Model file for the job. Use its own axes, mm. A direction names the side the tool comes from. Coordinates: 2 decimals unless noted, no trailing zeros. Write each loop counter-clockwise with the first axis right and the second up, starting at its lowest first coordinate (ties: lowest second). Pieces come first, ordered by that corner, then holes. Notation, with made-up numbers: M -36.5,27 L -22.5,27 A29 cw -22.5,64 Z; hole C 29.25,59 d4. An arc over 180 degrees is marked long. Put each result on its own line as item: value. Start each with the question number.
Q1. Which spindle directions (+Z, -Z, +X, -X, +Y, -Y) get a long thin tool onto all of the face, cutting with end or side? Do faces 1 (the flat face through (-58, -588, 85.706)), 2 (the flat face through (-38.133, -588, 26)), 3 (the flat face through (-80.633, -588, 26)). Say none if no direction does.
Q2. Pull direction Z, two halves, no side cores. Call faces 4 (the flat face through (-82.133, -588, 54)), 5 (the flat face through (-59, -588, -34.294)), 6 (the flat face through (-36.633, -588, 26)), 7 (the flat face through (-83.633, -588, 54)): pulls with the +Z half, pulls with the -Z half, needs draft (parallel to the pull), parting line crosses it, or undercut.
Q3. Drill centre lines: line 1 along X through (y, z) = (-846, 78.5); line 2 along X through (y, z) = (-259, 49); line 3 along Z through (x, y) = (-53.5, -513). Where is each one in solid material? Low to high.
Q4. Cut at A-A (x = -58.5). Write the cut outline in (y, z), then the cut area to 3 significant figures.
Q5. Drop flat-ended pins along their axis: pin 1 (5 mm diameter, centred on y = -998.5, z = -21.5, fed in from +X); pin 2 (4 mm diameter, centred on y = -742, z = 70.5, fed in from +X); pin 3 (19 mm diameter, centred on y = -639, z = 21, fed in from +X). Give the stop position or say it passes through.
```python
from build123d import *

# Parameters (mm, degrees)
F1_DEPTH = 1192
F2_T     = -1.5


with BuildPart() as f1:
    # F0 (on Front) → F1 (new body)
    with BuildSketch(Plane.XZ):
        with BuildLine():
            Line((-40.846474, 85.706456), (-76.418904, 85.706456))
            ThreePointArc((-76.418904, 85.706456), (-80.938799, 84.191483), (-83.632689, 80.258603))
            ThreePointArc((-83.632689, 80.258603), (-82.918779, 76.67027), (-80.88578, 73.628443))
            ThreePointArc((-80.88578, 73.628443), (-80.13546, 72.376035), (-80.065164, 70.917761))
            ThreePointArc((-80.065164, 70.917761), (-81.024186, 68.275196), (-82.723568, 66.035783))
            ThreePointArc((-82.723568, 66.035783), (-83.396078, 65.05222), (-83.632689, 63.884452))
            Line((-83.632689, 63.884452), (-83.632689, 42.902452))
            ThreePointArc((-83.632689, 42.902452), (-83.230765, 41.402452), (-82.132689, 40.304376))
            ThreePointArc((-82.132689, 40.304376), (-81.034613, 39.2063), (-80.632689, 37.7063))
            Line((-80.632689, 37.7063), (-80.632689, 13.706456))
            ThreePointArc((-80.632689, 13.706456), (-81.034613, 12.206456), (-82.132689, 11.10838))
            ThreePointArc((-82.132689, 11.10838), (-83.230765, 10.010304), (-83.632689, 8.510304))
            Line((-83.632689, 8.510304), (-83.632689, -10.388976))
            ThreePointArc((-83.632689, -10.388976), (-83.38823, -11.575142), (-82.694695, -12.567996))
            ThreePointArc((-82.694695, -12.567996), (-80.972966, -14.807673), (-80.030346, -17.470749))
            ThreePointArc((-80.030346, -17.470749), (-80.11711, -18.910604), (-80.865855, -20.143524))
            ThreePointArc((-80.865855, -20.143524), (-82.913386, -23.19222), (-83.632689, -26.793544))
            ThreePointArc((-83.632689, -26.793544), (-81.43599, -32.096845), (-76.132689, -34.293544))
            Line((-76.132689, -34.293544), (-41.132689, -34.293544))
            ThreePointArc((-41.132689, -34.293544), (-35.829388, -32.096845), (-33.632689, -26.793544))
            ThreePointArc((-33.632689, -26.793544), (-34.351992, -23.19222), (-36.399522, -20.143524))
            ThreePointArc((-36.399522, -20.143524), (-37.148267, -18.910604), (-37.235032, -17.470749))
            ThreePointArc((-37.235032, -17.470749), (-36.292412, -14.807673), (-34.570682, -12.567996))
            ThreePointArc((-34.570682, -12.567996), (-33.877147, -11.575142), (-33.632689, -10.388976))
            Line((-33.632689, -10.388976), (-33.632689, 8.510304))
            ThreePointArc((-33.632689, 8.510304), (-34.034613, 10.010304), (-35.132689, 11.10838))
            ThreePointArc((-35.132689, 11.10838), (-36.230765, 12.206456), (-36.632689, 13.706456))
            Line((-36.632689, 13.706456), (-36.632689, 37.7063))
            ThreePointArc((-36.632689, 37.7063), (-36.230765, 39.2063), (-35.132689, 40.304376))
            ThreePointArc((-35.132689, 40.304376), (-34.034613, 41.402452), (-33.632689, 42.902452))
            Line((-33.632689, 42.902452), (-33.632689, 63.884452))
            ThreePointArc((-33.632689, 63.884452), (-33.8693, 65.05222), (-34.541809, 66.035783))
            ThreePointArc((-34.541809, 66.035783), (-36.241192, 68.275196), (-37.200214, 70.917761))
            ThreePointArc((-37.200214, 70.917761), (-37.129917, 72.376035), (-36.379598, 73.628443))
            ThreePointArc((-36.379598, 73.628443), (-34.346598, 76.67027), (-33.632689, 80.258603))
            ThreePointArc((-33.632689, 80.258603), (-36.326579, 84.191483), (-40.846474, 85.706456))
        make_face()
    extrude(amount=F1_DEPTH)

    # F2
    f2_openings = [f1.faces().sort_by_distance(p)[0] for p in [
        (-58.632689, 0, 25.725749),
        (-58.632689, -1192, 25.725749),
    ]]
    offset(amount=F2_T, openings=f2_openings)


solid = f1.part
```
Computed values:
1. face 1: +Z, +X, -X, +Y, -Y
1. face 2: +Y, -Y
1. face 3: -X, +Y, -Y
2. face 4: undercut
2. face 5: pulls with the -Z half
2. face 6: undercut
2. face 7: needs draft
3. line 1: -83.47 to -81.93, -35.33 to -33.8
3. line 2: -83.63 to -82.13, -35.13 to -33.63
3. line 3: -34.29 to -32.79, 84.21 to 85.71
4. outline: M -1192,-34.29 L 0,-34.29 L 0,-32.79 L -1192,-32.79 Z; M -1192,84.21 L 0,84.21 L 0,85.71 L -1192,85.71 Z
4. area: 3,580 mm2
5. pin 1: x = -34.06
5. pin 2: x = -36.36
5. pin 3: x = -35.67
